Geometry: final body of the model. Coordinates: model frame, mm. Give positions to 0.01 mm unless a question says otherwise; leave off trailing zeros. Write each loop counter-clockwise with the first axis right and the second up, starting at its lowest first coordinate (ties: lowest second). Pieces come first, ordered by that corner, then holes. Notation, with made-up numbers: (50.5, -33) - (85.5, -33) arc R19 ccw to (85.5, -8) - close; hole circle Ø4 at (-18, -34). An arc over 180 degrees is marked (long way). Use CSV: the item, a comma, the result in double quotes. Start each with the question number.
(1) First-contact query: pin 1 Ø6 at (y, z) = (-0.5, 7.5) entering from +X; pin 2 Ø15.5 at (x, z) = (-249, 1.5) entering from -Y; pin 3 Ø1 at (x, z) = (-24.5, -1.5) entering from +Y. Flat tips, straight axial feed; report the tip coordinate or a pass-through.
(2) Section B-B on y = 24.5. Output: boundary loops of the cut face in (x, z).
(3) Section C-C on x = 186.5. Output: boundary loops of the cut face in (y, z), and give its area (3 significant figures).
(4) Line query: probe 1 along X at (y, z) = (-8, 0); probe 2 along X at (y, z) = (-4, -9); probe 3 along Y at (x, z) = (114.5, -4.5). Output: solid intervals per line, ascending. Write a range as [from, to].
(5) Section A-A on z = 0. Output: boundary loops of the cut face in (x, y).
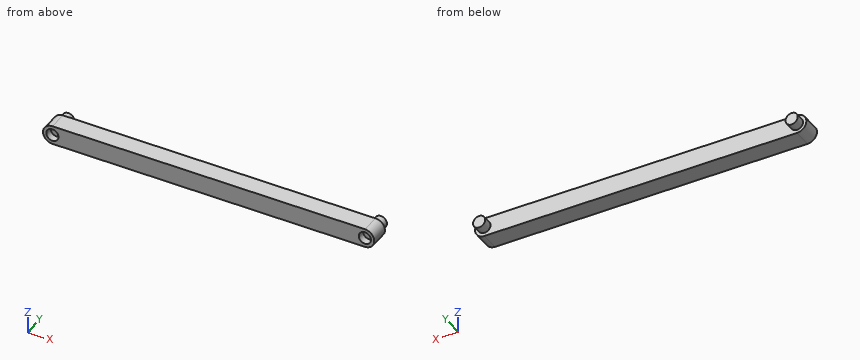
from build123d import *

# Parameters (mm, degrees)
BOSS_EXTRUDE1_DEPTH = 15
SKETCH2_R           = 9.75
BOSS_EXTRUDE2_DEPTH = 30
SKETCH2_2_R         = 9.75
CUT_EXTRUDE1_DEPTH  = 268.114207784
SKETCH2_3_R         = 9.75
BOSS_EXTRUDE3_DEPTH = 3


with BuildPart() as part:
    # Sketch1 → Boss-Extrude1 (new, symmetric)
    with BuildSketch(Plane(origin=(0, 0, 0), x_dir=(1, 0, 0), z_dir=(0, 1, 0))):
        with BuildLine():
            Line((-250, 15), (250, 15))
            ThreePointArc((250, 15), (265, 0), (250, -15))
            Line((250, -15), (-250, -15))
            ThreePointArc((-250, -15), (-265, 0), (-250, 15))
        make_face()
    extrude(amount=BOSS_EXTRUDE1_DEPTH, both=True)

    # Sketch2 → Boss-Extrude2 (add)
    with BuildSketch(Plane(origin=(0, 0, 0), x_dir=(1, 0, 0), z_dir=(0, 1, 0))):
        with Locations(Location((-250, 0, 0), (0, 0, 270))):
            Circle(SKETCH2_R)
        with Locations(Location((250, 0, 0), (0, 0, 270))):
            Circle(SKETCH2_R)
    extrude(amount=BOSS_EXTRUDE2_DEPTH)

    # Sketch2_2 → Cut-Extrude1 (cut, through all)
    with BuildSketch(Plane(origin=(0, 0, 0), x_dir=(1, 0, 0), z_dir=(0, 1, 0))):
        with Locations(Location((-250, 0, 0), (0, 0, 270))):
            Circle(SKETCH2_2_R)
        with Locations(Location((250, 0, 0), (0, 0, 270))):
            Circle(SKETCH2_2_R)
    extrude(amount=-CUT_EXTRUDE1_DEPTH, mode=Mode.SUBTRACT)

    # Sketch2_3 → Boss-Extrude3 (add)
    with BuildSketch(Plane(origin=(0, 0, 0), x_dir=(1, 0, 0), z_dir=(0, 1, 0))):
        with Locations(Location((-250, 0, 0), (0, 0, 270))):
            Circle(SKETCH2_3_R)
        with Locations(Location((250, 0, 0), (0, 0, 270))):
            Circle(SKETCH2_3_R)
    extrude(amount=-BOSS_EXTRUDE3_DEPTH)


solid = part.part
Check values:
1,pin 1,"stops at x = 264.31"
1,pin 2,"stops at y = -3"
1,pin 3,"stops at y = 15"
2,outline,"circle Ø19.5 at (-250, 0); circle Ø19.5 at (250, 0)"
3,outline,"(-15, -15) - (15, -15) - (15, 15) - (-15, 15) - close"
3,area,"900 mm²"
4,probe 1,"x = [-265, -259.75], [-240.25, 240.25], [259.75, 265]"
4,probe 2,"x = [-262, -253.75], [-246.25, 246.25], [253.75, 262]"
4,probe 3,"y = [-15, 15]"
5,outline,"(-265, -15) - (-259.75, -15) - (-259.75, -3) - (-240.25, -3) - (-240.25, -15) - (240.25, -15) - (240.25, -3) - (259.75, -3) - (259.75, -15) - (265, -15) - (265, 15) - (259.75, 15) - (259.75, 30) - (240.25, 30) - (240.25, 15) - (-240.25, 15) - (-240.25, 30) - (-259.75, 30) - (-259.75, 15) - (-265, 15) - close"
